Autodesk Inventor part; units mm, degrees
ref_plane "YZ Plane" through (0, 0, 0) normal (1, 0, 0) x (0, 1, 0)
ref_plane "XZ Plane" through (0, 0, 0) normal (0, 1, 0) x (-1, 0, 0)
ref_plane "XY Plane" through (0, 0, 0) normal (0, 0, 1) x (1, 0, 0)
sketch "スケッチ1" plane through (0, 0, 0) normal (0, 1, 0) x (-1, 0, 0)
  circle A0 centre (0, 0) radius 35
  line L0 (0, 0) -> (0, -35)
  line L1 (0, 0) -> (0, 35)
  dimension "d0" = 70
revolve "回転1" add sketch "スケッチ1" angle 180 about axis through (0, 0, 0) along (0, 0, 1) picked at (-2.5961, -23.0408) contours L1 L0 A0
sketch "スケッチ5" plane through (0, 0, 0) normal (0, -1, 0) x (1, 0, 0)
  line L0 (-20, -25) -> (20, -25)
  line L1 (20, -25) -> (20, -18)
  line L2 (20, -18) -> (-20, -18)
  line L3 (-20, -18) -> (-20, -25)
  line L4 (-20, -18) -> (-23, -18)
  line L5 (-23, -18) -> (-23, -20)
  line L6 (-23, -20) -> (-20, -20)
  line L7 (-20, -20) -> (-20, -18)
  line L8 (0, 26.2) -> (-17, 26.2)
  line L9 (-17, 26.2) -> (-17, 25)
  line L10 (-17, 25) -> (0, 25)
  line L11 (0, 25) -> (0, 26.2)
  line L12 (0, 21) -> (-20, 21)
  line L13 (-20, 21) -> (-20, 20)
  line L14 (-20, 20) -> (0, 20)
  line L15 (0, 20) -> (0, 21)
  line L16 (0, 13) -> (-19, 13)
  line L17 (-19, 13) -> (-19, 11.4)
  line L18 (-19, 11.4) -> (0, 11.4)
  line L19 (0, 11.4) -> (0, 13)
  line L20 (0, 4.4) -> (-20, 4.4)
  line L21 (-20, 4.4) -> (-20, 3.4)
  line L22 (-20, 3.4) -> (0, 3.4)
  line L23 (0, 3.4) -> (0, 4.4)
  circle A0 centre (0, 0) radius 35
  circle A1 centre (0, 0) radius 35
  line L24 (0, 35) -> (0, -35)
  line L25 (35, 0) -> (-35, 0)
  line L26 (-31.236, 1.9738) -> (-22.236, 1.9738)
  line L27 (-22.236, 1.9738) -> (-22.236, -8.0262)
  line L28 (-22.236, -8.0262) -> (-31.236, -8.0262)
  line L29 (-31.236, -8.0262) -> (-31.236, 1.9738)
  line L30 (-22.236, 1.9738) -> (-7.236, 1.9738)
  line L31 (-7.236, 1.9738) -> (-7.236, -8.0262)
  line L32 (-7.236, -8.0262) -> (-22.236, -8.0262)
  line L33 (-22.236, -8.0262) -> (-22.236, 1.9738)
  line L34 (-27, 22.2711) -> (-27, -22.2711)
  line L35 (-20.736, 3.4738) -> (-32.736, 3.4738)
  line L36 (-32.736, 3.4738) -> (-32.736, -9.5262)
  line L37 (-32.736, -9.5262) -> (-20.736, -9.5262)
  line L38 (-20.736, -9.5262) -> (-20.736, 3.4738)
  line L39 (-20.736, 3.4738) -> (-32.736, -9.5262) construction
  line L40 (-32.736, 3.4738) -> (-20.736, -9.5262) construction
  line L41 (-16, 26.2) -> (0, 26.2)
  line L42 (0, 26.2) -> (0, 35)
  line L43 (0, 35) -> (-16, 35)
  line L44 (-16, 35) -> (-16, 26.2)
  line L45 (-16, 25) -> (0, 25)
  line L46 (0, 25) -> (0, 22)
  line L47 (0, 22) -> (-16, 22)
  line L48 (-16, 22) -> (-16, 25)
  line L49 (-18, 13) -> (0, 13)
  line L50 (0, 13) -> (0, 19)
  line L51 (0, 19) -> (-18, 19)
  line L52 (-18, 19) -> (-18, 13)
  line L53 (-18, 11.4) -> (0, 11.4)
  line L54 (0, 11.4) -> (0, 5.4)
  line L55 (0, 5.4) -> (-18, 5.4)
  line L56 (-18, 5.4) -> (-18, 11.4)
  line L57 (-22.236, -3.0262) -> (-37.4009, -3.0262)
  point P0 (0, -25)
  point P1 (0, -18)
  point P2 (-20, -20)
  point P3 (0, 25.6)
  point P4 (0, 20.5)
  point P5 (0, 12.2)
  point P6 (0, 3.9)
  point P7 (-20, -21.5)
  point P8 (-27, 1.9738)
  point P9 (-27, -8.0262)
  point P10 (-26.736, -3.0262)
  point P11 (-16, 23.5)
  point P12 (-16, 31.1288)
  point P13 (0, 25)
  point P14 (0, 11.4)
  dimension "d12" = 40
  dimension "d13" = 7
  dimension "d21" = 3
  dimension "d22" = 2
  dimension "d23" = 17
  dimension "d24" = 1.2
  dimension "d27" = 20
  dimension "d28" = 1
  dimension "d30" = 19
  dimension "d31" = 1.6
  dimension "d33" = 1
  dimension "d88" = 0
  dimension "d89" = 0
  dimension "d90" = 10
  dimension "d92" = 20
  dimension "d93" = 8.8
  dimension "d94" = 14
  dimension "d95" = 22
  dimension "d96" = 30.6
  dimension "d97" = 9
  dimension "d98" = 10
  dimension "d99" = 1.4262
  dimension "d100" = 2.236
  dimension "d101" = 15
  dimension "d102" = 9.9738
  dimension "d113" = 27
  dimension "d116" = 12
  dimension "d117" = 13
  dimension "d120" = 0.0738
  dimension "d121" = 0.736
  dimension "d122" = 16
  dimension "d123" = 35
  dimension "d124" = 3
  dimension "d125" = 16
  dimension "d126" = 6
  dimension "d127" = 6
  dimension "d128" = 18
  dimension "d129" = 18
extrude "GNSボード" cut sketch "スケッチ5" against normal blind 16 contours L11 L10 L9 L8
extrude "GNSボード止めるよう" cut sketch "スケッチ5" against normal blind 15 contours L24 L8 L44 A0 | L24 L47 L48 L10
extrude "アルミ板１" cut sketch "スケッチ5" against normal blind 20 contours L15 L14 L13 L12
extrude "メイン基板" cut sketch "スケッチ5" against normal blind 17.5 contours L18 L17 L16 L19
extrude "メイン止めるよう" cut sketch "スケッチ5" against normal blind 16.5 contours L55 L56 L18 L24 | L16 L52 L51 L24
extrude "アルミ板２" cut sketch "スケッチ5" against normal blind 17.5 contours L22 L21 L20 L23
extrude "モーター" cut sketch "スケッチ5" against normal blind 6 contours L31 L32 L38 L25 | L25 L38 L30 L31 | L38 L32 L27 L25 | L25 L27 L30 L38 | L34 L57 L27 L28 | L28 L29 L57 L34 | L27 L57 L34 L25 | L25 L34 L26 L27 | L29 L25 L34 L57 | L25 L29 L26 L34
extrude "モーター受け" add sketch "スケッチ5" against normal blind 9 contours L37 L36 L57 L29 L28 L34 | L34 L28 L32 L38 L37 | L38 L32 L27 L25 | L25 L27 L30 L38 | L36 L25 L29 L57 | L34 L57 L27 L28 | L28 L29 L57 L34 | L27 L57 L34 L25 | L25 L34 L26 L27 | L30 L26 L34 L35 L38 | L36 L35 L34 L26 L29 L25 | L29 L25 L34 L57 | L25 L29 L26 L34
extrude "電池ボックス入れ" cut sketch "スケッチ5" against normal blind 15 contours L3 L2 L24 L0 | L24 L2 L1 L0 | L6 L5 L4 L3
extrude "サイドかっと" cut sketch "スケッチ5" against normal blind 1 contours A0 L57 L36 L37 L34 | A0 L25 L36 L57 | L37 L36 L57 L29 L28 L34 | A0 L34 L35 L36 L25 | L36 L25 L29 L57 | L36 L35 L34 L26 L29 L25
ref_plane "作業平面3" through (-32.736, 9, -9.5262) normal (-1, 0, 0) x (0, 0, -1)
sketch "スケッチ23" plane through (-32.736, 9, -9.5262) normal (-1, 0, 0) x (0, 0, -1)
  line L0 (-11.5, 9) -> (-1.5, 9)
  circle A0 centre (-6.5, 9) radius 2.5
  point P0 (-9.5262, 9)
  dimension "d134" = 5
extrude "押し出し21" cut sketch "スケッチ23" against normal blind 2
properties part number "naibu"
Geometry: final body of the model. Coordinates: model frame, mm. A direction names the side the tool comes from. Give positions to 0.01 mm unless a question says otherwise; leave off trailing zeros. Write each loop counter-clockwise with the first axis right and the second up, starting at its lowest first coordinate (ties: lowest second). Pieces come first, ordered by that corner, then holes.
(1) Cut plane B-B, the plane x = 9. Return loops of the section in (y, z), then the cut area to 3 significant figures.
(2) First-contact query: P1, Ø3, axis at x = -10.5, z = 7, coming from the -Y side; P2, Ø16, axis at x = -10.5, y = 5.5, coming from the -Z side; P3, Ø5, axis at x = -8, y = 18.5, coming from the +Z side. Flat tips, straight axial feed; report the tip coordinate or a pass-through.
(3) Cut plane C-C, the plane y = 24. Return loops of the section in (x, z), then the cut area to 3 significant figures.
(4) Ray query, line 1 (Z direction, x = -15.5, y = 4.5); line 2 (Z direction, x = 17, y = 8); line 3 (X direction, y = 2.5, z = 9.5). Return the intervals inside material, ascending.
(5) Mould query, pull axis Z, two halves, no side actions, for faces 3 (the flat face through (-32, 1, 0)), 4 (the flat face through (-14, 6, -3)). Classes: released by +Z, released by -Z, zero draft, split by the parting line, or undercut.
(6) Cut plane D-D, the plane x = -6. Return loops of the section in (y, z), then the cut area to 3 significant figures.
(7) Access query for faces 1 (the flat face through (-1, 7, -18)), 2 (the flat face through (-16, 7, 23)). Directions: +Z, -Z, +X, -X, +Y, -Y. A direction counts if a zero-diameter tool reaches every point of the face in a straight line with its end or side. Return the directions, or none.
Values follow:
1. outline: (0, -33.82) arc R33.82 ccw to (0, 33.82) - (0, -18) - (15, -18) - (15, -25) - (0, -25) - close
1. area: 1,690 mm2
2. P1: stops at y = 16.5
2. P2: stops at z = -34.79
2. P3: stops at z = 30.22
3. outline: circle Ø50.95 at (0, 0)
3. area: 2,040 mm2
4. line 1: z = -31.06 to -25, -18 to -8.03, 1.97 to 3.4, 4.4 to 5.4, 19 to 20, 21 to 22
4. line 2: z = -29.53 to -25, -18 to 29.53
4. line 3: x = -33.59 to -18, 0 to 33.59
5. face 3: zero draft
5. face 4: undercut
6. outline: (0, -34.48) arc R34.48 ccw to (15, 31.05) - (15, 26.2) - (16, 26.2) - (16, 25) - (15, 25) - (15, 22) - (0, 22) - (0, 21) - (20, 21) - (20, 20) - (0, 20) - (0, 19) - (16.5, 19) - (16.5, 13) - (17.5, 13) - (17.5, 11.4) - (16.5, 11.4) - (16.5, 5.4) - (0, 5.4) - (0, 4.4) - (17.5, 4.4) - (17.5, 3.4) - (0, 3.4) - (0, -18) - (15, -18) - (15, -25) - (0, -25) - close
6. area: 1,330 mm2
7. face 1: -Y
7. face 2: +Z, -Y
